Part model, mm, in its own coordinate system. A direction names the side the tool comes from. Give positions to 0.01 mm unless a question says otherwise; leave off trailing zeros. Write each loop counter-clockwise with the first axis right and the second up, starting at its lowest first coordinate (ties: lowest second). Pieces come first, ordered by that corner, then holes.
Autodesk Fusion 360 part; units mm, degrees
sketch "Sketch1" plane through (0, 0, 0) normal (0, 1, 0) x (1, 0, 0)
  line L0 (11.3137, 14) -> (32, 14)
  line L1 (32, 14) -> (32, -14)
  line L2 (32, -14) -> (11.3137, -14)
  arc A0 (11.3137, 14) -> (11.3137, -14) centre (0, 0) ccw
  line L3 (32, -12.5) -> (10.7703, -12.5)
  arc A1 (10.7703, 12.5) -> (10.7703, -12.5) centre (0, 0) ccw
  line L4 (10.7703, 12.5) -> (32, 12.5)
  circle A2 centre (0, 0) radius 2.75
  dimension "d1" = 36
  dimension "d4" = 1.5
  dimension "d5" = 5.5
extrude "Extrude1" add sketch "Sketch1" along normal blind 40 contours L0 L1 L2 A0 L3 A1 L4 | L1 L3 A1 L4 | A2
extrude "Extrude2" cut sketch "Sketch1" along normal through all from surface at 1.5 contours L1 L3 A1 L4 | A2
extrude "Extrude3" add sketch "Sketch1" against normal blind 4 contours A2
sketch "Sketch2" plane through (0, 0, 0) normal (0, 0, 1) x (1, 0, 0)
  line L0 (15.3745, -4.2511) -> (35, 35)
  line L1 (35, 35) -> (35, 42)
  line L2 (35, 42) -> (8, 42)
  line L3 (8, 42) -> (-19, 5)
  line L4 (-19, 5) -> (-19, -4.2511)
  line L5 (-19, -4.2511) -> (15.3745, -4.2511)
  circle A0 centre (25, 34) radius 2.5
  dimension "d12" = 5
extrude "Extrude4" cut sketch "Sketch2" along normal through all and the other way through all keep common part
1) 3-axis set-ups, long thin cutter, end or side, ignore diameter. For faces 1 (the flat face through (32, 34, 13)), 2 (the flat face through (19, 25, -12.5)), 3 (the flat face through (19, 24, -14)), 4 (the flat face through (20, 24, 14)), 5 (the cylindrical face through (-8.265, 16.203, 14.281)): which of +Z, -Z, +X, -X, +Y, -Y reach the whole face in a straight line?
Check result:
face 1: +Z, -Z, +X, +Y, -Y
face 2: +X, +Y
face 3: -Z, +X, +Y, -Y
face 4: +Z, +X, +Y, -Y
face 5: +Y
2) Saw through at B-B (y = 28). Write the cut outline in (x, z).
Check result:
outline: (-2.22, -17.86) arc R18 ccw to (11.31, -14) - (31.5, -14) - (31.5, -12.5) - (10.77, -12.5) arc R16.5 cw to (-2.22, -16.35) - close; (-2.22, 16.35) arc R16.5 cw to (10.77, 12.5) - (31.5, 12.5) - (31.5, 14) - (11.31, 14) arc R18 ccw to (-2.22, 17.86) - close
3) Saw through at A-A (x = 25). Write the cut outline in (y, z).
Check result:
outline: (15, -14) - (31.5, -14) - (31.5, -12.5) - (15, -12.5) - close; (15, 12.5) - (31.5, 12.5) - (31.5, 14) - (15, 14) - close; (36.5, -14) - (40, -14) - (40, -12.5) - (36.5, -12.5) - close; (36.5, 12.5) - (40, 12.5) - (40, 14) - (36.5, 14) - close
4) Drill centre lines: L1, parallel to Z at x = 0, y = 19.5; L2, parallel to Z at x = 16.5, y = 29.5; L3, parallel to Y at x = -7.5, z = 4.5. Where is each one in solid material? Low to high.
Check result:
L1: z = -18 to -16.5, 16.5 to 18
L2: z = -14 to -12.5, 12.5 to 14
L3: y = 0 to 1.5
5) Flat gauge pins, fed straight in: P1, Ø6, axis at x = 23, y = 17.5, coming from the -Z side; P2, Ø1.5, axis at y = 7.5, z = -4.5, coming from the -X side; P3, Ø3, axis at x = 2, y = 13, coming from the -Z side. Where does each tip first touch, or does it go through?
Check result:
P1: stops at z = -14
P2: stops at x = -17.56
P3: stops at z = -17.99
6) Saw through at C-C (z = 0). Write the cut outline in (x, y).
Check result:
outline: (-18, 0) - (-2.75, 0) - (-2.75, -4) - (2.75, -4) - (2.75, 0) - (17.5, 0) - (18.25, 1.5) - (-16.5, 1.5) - (-16.5, 8.43) - (-18, 6.37) - close
7) Saw through at D-D (y = 34). Write the cut outline in (x, z), and give its area (3 significant figures).
Check result:
outline: (2.16, -17.87) arc R18 ccw to (11.31, -14) - (22.5, -14) - (22.5, -12.5) - (10.77, -12.5) arc R16.5 cw to (2.16, -16.36) - close; (2.16, 16.36) arc R16.5 cw to (10.77, 12.5) - (22.5, 12.5) - (22.5, 14) - (11.31, 14) arc R18 ccw to (2.16, 17.87) - close; (27.5, -14) - (32, -14) - (32, -12.5) - (27.5, -12.5) - close; (27.5, 12.5) - (32, 12.5) - (32, 14) - (27.5, 14) - close
area: 77.3 mm2
8) Mould opens along Y. For faces 6 (the cylindrical face through (-0.596, -1.972, 2.685)), 7 (the cylindrical face through (23.16, 32.31, -13.26)), 8 (the flat face through (3, 0, 0)), 9 (the cylindrical face through (23.16, 32.31, 13.24)) say: +Y half, -Y half, draft (parallel to the pull), parting line (faces both ways), or undercut.
Check result:
face 6: draft
face 7: undercut
face 8: -Y half
face 9: undercut
